The figure shows three views and two pictorial views of one solid part (mm, origin at its lowest corner). Answer the questions. Round coordinates to 2 decimals unless told otherwise and drop trailing zeros. Order: outer loops, then holes, each group sorted by start corner. A loop starts at its lowest first (then second) coordinate and runs counter-clockwise, first axis right, second up. Notation, with made-up numbers: (-9, 37.25) -> (32, 37.25) arc R15 cw to (32, 51.25) -> close; hole circle Ø10 at (54, 0). An arc over 180 degrees is marked (long way). One line per item, written item: value. Start each with the question number.
1. Section C-C (z = 21.5) is taken. Give the vertices of the cut face in (x, y), then the cut area to 3 significant figures.
2. Section A-A (z = 48) is taken. Give the vertices of the cut face in (x, y), then the cut area to 3 significant figures.
3. A flat-ended cylindrical pin translates along its axis: pin 1 Ø0.6 at (y, z) = (0.5, 40) entering from -X. Find the tip coordinate at first contact, or state that the pin passes through.
4. Consider line 1 (X direction, y = 1.8, z = 41.5); line 2 (X direction, y = 0.2, z = 19); line 3 (Z direction, x = 38.5, y = 0.15). Determine where each line is inside the solid, lowest interval first.
5. Section D-D (y = 0.95) is taken. State how many separate pieces and enclosed holes the cut face has, then the cut area to 3 significant figures.
6. Section B-B (x = 34) is taken. Give the vertices of the cut face in (y, z).
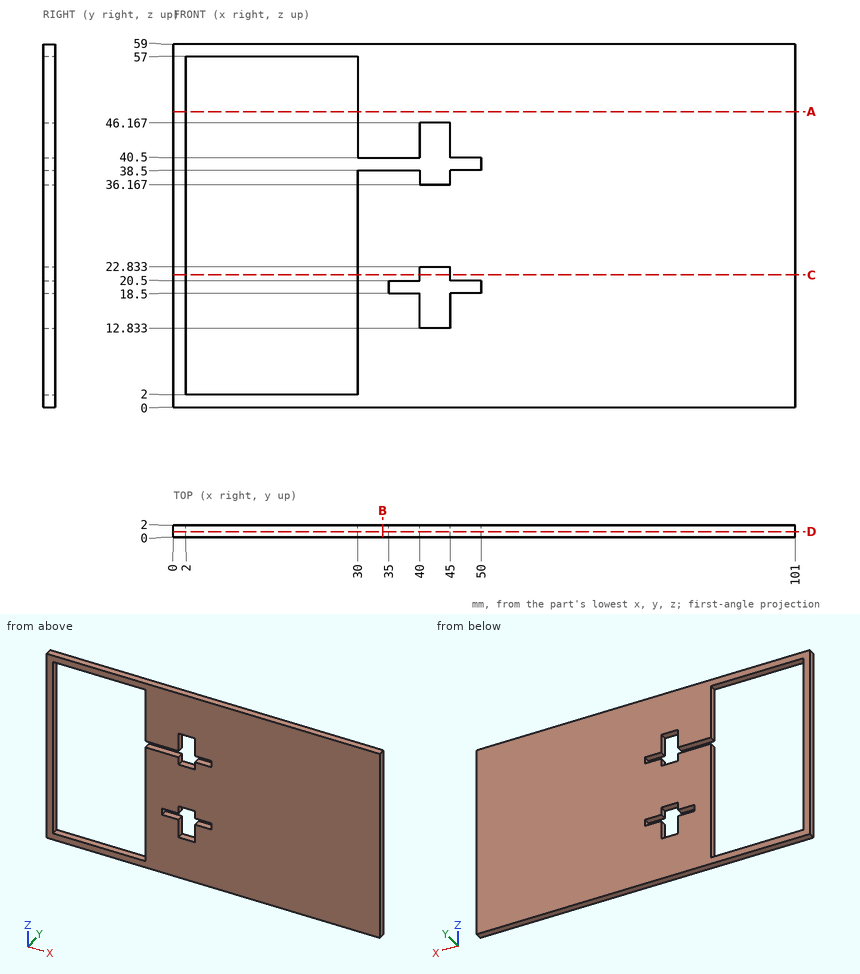
Answer:
1. outline: (0, 0) -> (2, 0) -> (2, 2) -> (0, 2) -> close; (30, 0) -> (40, 0) -> (40, 2) -> (30, 2) -> close; (45, 0) -> (101, 0) -> (101, 2) -> (45, 2) -> close
1. area: 136 mm^2
2. outline: (0, 0) -> (2, 0) -> (2, 2) -> (0, 2) -> close; (30, 0) -> (101, 0) -> (101, 2) -> (30, 2) -> close
2. area: 146 mm^2
3. pin 1: x = 0
4. line 1: 0 to 2, 30 to 40, 45 to 101
4. line 2: 0 to 2, 30 to 35, 50 to 101
4. line 3: 0 to 18.5, 20.5 to 38.5, 40.5 to 59
5. separate pieces: 1
5. enclosed holes: 2
5. area: 4,270 mm^2
6. outline: (0, 0) -> (2, 0) -> (2, 38.5) -> (0, 38.5) -> close; (0, 40.5) -> (2, 40.5) -> (2, 59) -> (0, 59) -> close
